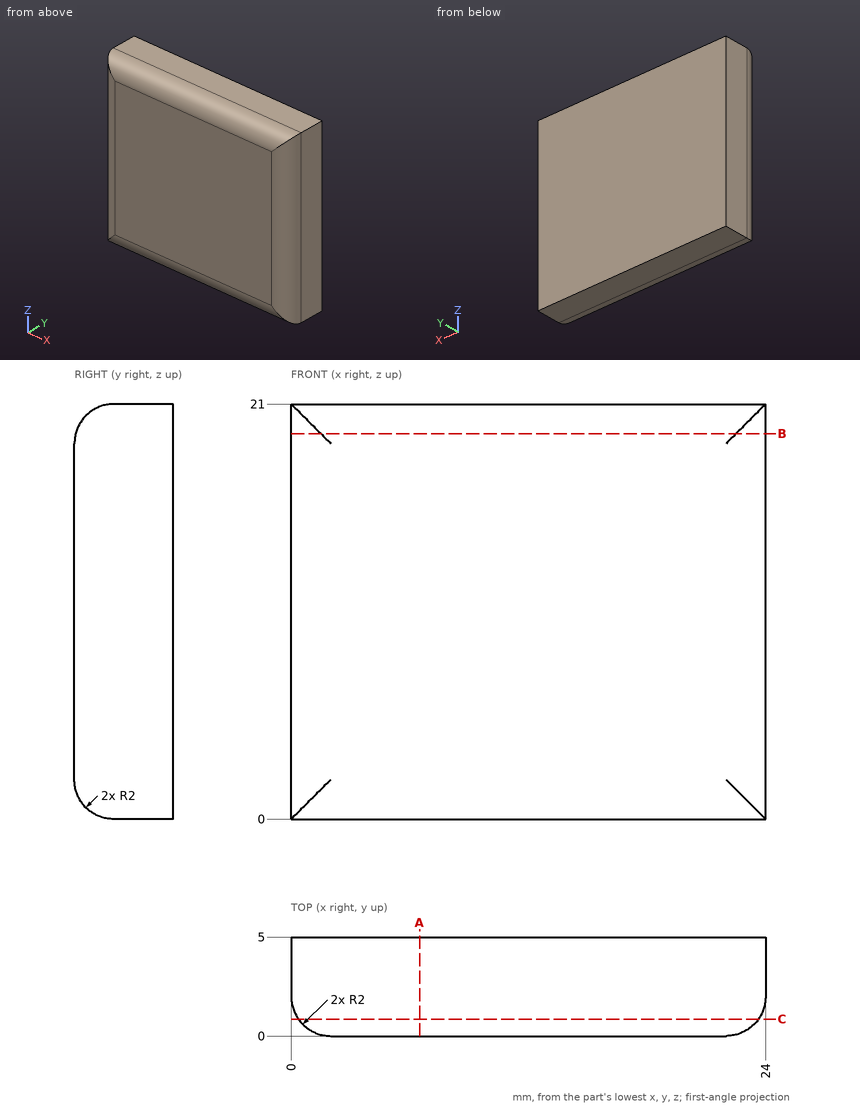
Could you check a few things on this drawing? It's one solid part, dimensions in mm from its lowest x, y, z. Round coordinates to 2 decimals unless told otherwise and drop trailing zeros. Write each loop counter-clockwise with the first axis right and the second up, starting at its lowest first coordinate (ties: lowest second). Pieces come first, ordered by that corner, then holes. Notation, with made-up numbers: (-27, 47) -> (7, 47) arc R26 ccw to (7, 61) -> close; hole circle Ø1 at (43, -21). An arc over 180 degrees is marked (long way). Use one line per item in the form item = value. Start each with the question number.
Q1. Imagine slicing it at A-A (x = 6.5). Please give me the cut outline in (y, z), then the cut area to 3 significant figures.
Q2. Imagine slicing it at B-B (z = 19.5). Please give me the cut outline in (x, y), then the cut area to 3 significant figures.
Q3. If I drill on probe 1 along Z at (x, y) = (12.5, 1.85); probe 2 along X at (y, z) = (1.1, 4); probe 3 along Z at (x, y) = (17.5, 1), over which ranges is the centre line in solid material (lowest first)? Write a range as [from, to].
Q4. I'm going to push a flat-ended pin straight in: P1, Ø3, axis at y = 3.5, z = 13.5, coming from the -X side. Where does the tip first touch, or does it pass through?
Q5. Imagine slicing it at C-C (y = 0.85). Please give me the cut outline in (x, z).
Worked out:
q1.outline = (0, 2) arc R2 ccw to (2, 0) -> (5, 0) -> (5, 21) -> (2, 21) arc R2 ccw to (0, 19) -> close
q1.area = 103 mm^2
q2.outline = (0, 2) arc R2 ccw to (1.5, 0.06) -> (22.5, 0.06) arc R2 ccw to (24, 2) -> (24, 5) -> (0, 5) -> close
q2.area = 117 mm^2
q3.probe_1 = [0.01, 20.99]
q3.probe_2 = [0.21, 23.79]
q3.probe_3 = [0.27, 20.73]
q4.P1 = 0
q5.outline = (0.36, 0.36) -> (23.64, 0.36) -> (23.64, 20.64) -> (0.36, 20.64) -> close
